from build123d import *

# Parameters (mm, degrees)
FILLET1_R     = 3.175
CHAMFER1_SIZE = 0.762
FILLET2_R     = 2.54


with BuildPart() as part:
    # Sketch3 → Revolve1 (revolve)
    with BuildSketch(Plane.XY):
        Polygon((-34.629025424, 22.543396893), (-13.991525424, 22.543396893), (-13.991525424, 17.780896893), (-28.977525424, 17.780896893), (-28.977525424, 5.080896893), (-31.263525424, 5.080896893), (-31.263525424, 17.780896893), (-34.629025424, 17.780896893), align=None)
    revolve(axis=Axis((-13.991525424, 22.543396893, 0), (0, -1, 0)))

    # Fillet1
    fillet1_edges = [part.edges().sort_by_distance(p)[0] for p in [
        (6.645974576, 22.543396893, 0),
    ]]
    fillet(fillet1_edges, radius=FILLET1_R)

    # Chamfer1
    chamfer1_edges = [part.edges().sort_by_distance(p)[0] for p in [
        (3.280474576, 17.780896893, 0),
        (3.280474576, 5.080896893, 0),
    ]]
    chamfer(chamfer1_edges, length=CHAMFER1_SIZE)

    # Fillet2
    fillet2_edges = [part.edges().sort_by_distance(p)[0] for p in [
        (0.994474576, 17.780896893, 0),
    ]]
    fillet(fillet2_edges, radius=FILLET2_R)


solid = part.part
CAD build for the part. Positions are in the model's coordinates, mm. A direction names the side the tool comes from. Round coordinates to 2 decimals unless told otherwise and drop trailing zeros. Loops run counter-clockwise (first coordinate to the right, second up) from the corner with the lowest first, then second, coordinate; pieces in that order, holes last. Notation, with made-up numbers: M -17.5,-23.5 L -8.5,-23.5 A20 ccw -8.5,4.5 Z; hole C -3.75,-40 d4. An arc over 180 degrees is marked long. One line per question, with ' | ' between items. Start each with the question number.
Item 1: Cut at A-A, the plane z = 0. Write the cut outline in (x, y) (3 decimals), plus the area to 3 significant figures.
Item 2: Pin check, flat tips, straight feed: pin 1 Ø20 at (x, z) = (-14, -2.5) entering from -Y; pin 2 Ø4 at (x, y) = (-30.5, 16.5) entering from -Z; pin 3 Ø8 at (x, y) = (-27, 10) entering from +Z. Stop position of each tip, or through.
Item 3: Which spindle directions (+Z, -Z, +X, -X, +Y, -Y) get a long thin tool onto all of the face, cutting with end or side? Do faces 4 (the flat face through (-10, 5.081, 15)), 5 (the cylindrical face through (-11.743, 11.509, -17.125)). Say none if no direction does.
Item 4: Cut at B-B, the plane y = 7.5. Write the cut outline in (x, z).
Item 5: Cut at C-C, the plane y = 15.75. Write the cut outline in (x, z).
Item 6: Two-plate mould, pull along X, no slides. Class faces 1 (the flat face through (-14, 17.781, 0)), 2 (the cylindrical face through (-33.055, 18.586, 7.904)), 3 (the flat face through (-14.1, 17.781, 18.2)): pulls with the +X half, pulls with the -X half, needs draft (parallel to the pull), parting line crosses it, or undercut.
Item 7: Wall check: line 1 (Z direction, x = -14.5, y = 10); line 2 (X direction, y = 11.75, z = 0); line 3 (Y direction, x = -8.5, z = 10). Give the ranges that are in metal, low to high.
Responses:
1) outline: M -34.629,17.781 L -32.026,17.781 L -31.264,17.019 L -31.264,5.843 L -30.502,5.081 L -28.978,5.081 L -28.978,15.241 A2.54 cw -26.438,17.781 L -1.546,17.781 A2.54 cw 0.994,15.241 L 0.994,5.081 L 2.518,5.081 L 3.28,5.843 L 3.28,17.019 L 4.042,17.781 L 6.646,17.781 L 6.646,19.368 A3.175 ccw 3.471,22.543 L -31.454,22.543 A3.175 ccw -34.629,19.368 Z | area: 253 mm²
2) pin 1: stops at y = 17.78 | pin 2: stops at z = -14.2 | pin 3: stops at z = 14.74
3) face 4: +Z, -Z, +X, -X, -Y | face 5: -Y
4) outline: C -13.99,0 d34.54; hole C -13.99,0 d29.97
5) outline: C -13.99,0 d34.54; hole C -13.99,0 d29.87
6) face 1: undercut | face 2: parting line crosses it | face 3: needs draft
7) line 1: z = -17.26 to -14.98, 14.98 to 17.26 | line 2: x = -31.26 to -28.98, 0.99 to 3.28 | line 3: y = 17.78 to 22.54
